Verification items for the finished model (mm, model axes). Face numbers are marked on the shaded views. A direction names the side the tool comes from. Round coordinates to 2 decimals unless told otherwise and drop trailing zeros. Write each loop counter-clockwise with the first axis right and the second up, starting at its lowest first coordinate (ties: lowest second). Pieces come first, ordered by that corner, then holes. Notation, with made-up numbers: M 19,83.25 L 71,83.25 A20 ccw 71,89.25 Z; hole C -14.75,44 d5. An arc over 180 degrees is marked long. One line per item, written item: value. Start each with the question number.
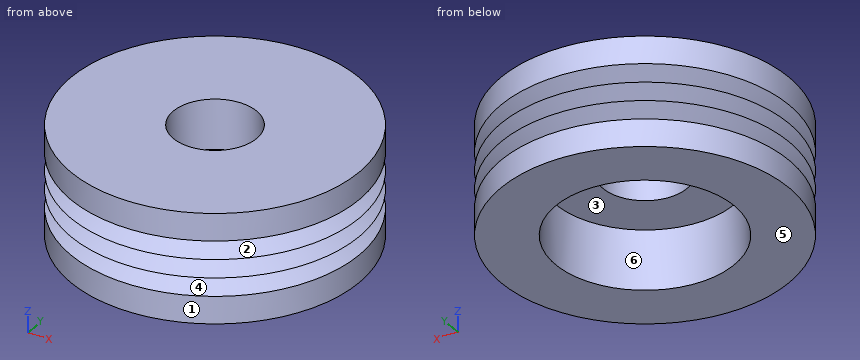
from build123d import *

# Parameters (mm, degrees)
SKETCH3_R          = 4.5
CUT_EXTRUDE1_DEPTH = 3
SKETCH4_R          = 2.1
CUT_EXTRUDE2_DEPTH = 11.68293031


with BuildPart() as part:
    # Sketch2 → Revolve1 (revolve)
    with BuildSketch(Plane(origin=(0, 0, 0), x_dir=(1, 0, 0), z_dir=(0, 1, 0))):
        Polygon((0, 5.5), (-7.25, 5.5), (-7.25, 4.127624556), (-6.25, 3.666666667), (-7.25, 3.210957889), (-6.25, 2.755249111), (-7.25, 2.294291222), (-6.25, 1.833333333), (-7.25, 1.372375444), (-7.25, 0), (0, 0), align=None)
    revolve(axis=Axis((0, 0, -5.5), (0, 0, 1)))

    # Sketch3 → Cut-Extrude1 (cut)
    with BuildSketch(Plane(origin=(0, 0, -5.5), x_dir=(-1, 0, 0), z_dir=(0, 0, -1))):
        Circle(SKETCH3_R)
    extrude(amount=-CUT_EXTRUDE1_DEPTH, mode=Mode.SUBTRACT)

    # Sketch4 → Cut-Extrude2 (cut, through all)
    with BuildSketch(Plane(origin=(0, 0, -2.5), x_dir=(-1, 0, 0), z_dir=(0, 0, -1))):
        Circle(SKETCH4_R)
    extrude(amount=-CUT_EXTRUDE2_DEPTH, mode=Mode.SUBTRACT)


solid = part.part
1) Cross-section at D-D (z = -0.95). Record the boundary of the cut face in (x, y), then the cut area to 3 significant figures.
2) Cross-section at C-C (z = -4.95). Record the boundary of the cut face in (x, y), then the cut area to 3 significant figures.
3) Mould release check, pull along Z, two halves, no side actions. Record for the marked faces 4, 5 and 6: pulls with the +Z half, pulls with the -Z half, needs draft (parallel to the pull), parting line crosses it, or undercut.
4) Gauge pin test, flat ends, axial feed: pin 1 Ø4.5 at (x, y) = (0, -0.5) entering from -Z; pin 2 Ø2 at (x, z) = (5, -4.5) entering from -Y; pin 3 Ø7 at (x, y) = (0, 0) entering from +Z; pin 4 Ø1 at (x, z) = (1, -1.5) entering from +Y. Record the tip position at first contact, or that the pin passes through.
5) Access from +Z, -Z, +X, -X, +Y, -Y to the whole of each face (thin tool, end or side, straight path). Record for the marked faces 1, 2 and 3.
6) Cross-section at A-A (y = 0). Record the boundary of the cut face in (x, z).
7) Thickness scan on line 1 (Y direction, x = 0, z = -0.9); line 2 (X direction, y = 0.75, z = -1.3); line 3 (X direction, y = -4, z = -4.75). Record the ranges inside material, lowest first.
Results below:
1. outline: C 0,0 d14.5; hole C 0,0 d4.2
1. area: 151 mm²
2. outline: C 0,0 d14.5; hole C 0,0 d9
2. area: 102 mm²
3. face 4: undercut
3. face 5: pulls with the -Z half
3. face 6: needs draft
4. pin 1: stops at z = -2.5
4. pin 2: stops at y = -6.05
4. pin 3: stops at z = 0
4. pin 4: stops at y = 7.23
5. face 1: +Z, -Z
5. face 2: none
5. face 3: -Z
6. outline: M -7.25,-5.5 L -4.5,-5.5 L -4.5,-2.5 L -2.1,-2.5 L -2.1,0 L -7.25,0 L -7.25,-1.37 L -6.25,-1.83 L -7.25,-2.29 L -6.25,-2.76 L -7.25,-3.21 L -6.25,-3.67 L -7.25,-4.13 Z; M 2.1,-2.5 L 4.5,-2.5 L 4.5,-5.5 L 7.25,-5.5 L 7.25,-4.13 L 6.25,-3.67 L 7.25,-3.21 L 6.25,-2.76 L 7.25,-2.29 L 6.25,-1.83 L 7.25,-1.37 L 7.25,0 L 2.1,0 Z
7. line 1: y = -7.25 to -2.1, 2.1 to 7.25
7. line 2: x = -7.21 to -1.96, 1.96 to 7.21
7. line 3: x = -6.05 to -2.06, 2.06 to 6.05
